from build123d import *

# Parameters (mm, degrees)
SKETCH1_W               = 24.51
SKETCH1_H               = 148
BOSS_EXTRUDE1_DEPTH     = 8
SKETCH2_W               = 8
SKETCH2_H               = 148
BOSS_EXTRUDE2_DEPTH     = 25
SKETCH4_W               = 20.3
SKETCH4_H               = 36.8
BOSS_EXTRUDE3_DEPTH     = 8
SKETCH5_W               = 23
SKETCH5_H               = 6
BOSS_EXTRUDE4_DEPTH     = 25
CUT_EXTRUDE2_REACH      = 151.752
SKETCH6_R               = 2
RIB1_REACH              = 159.03
SKETCH8_WALL_W          = 336.456302216
SKETCH8_WALL_H          = 3
MIRROR2_COPY_1_REACH    = 159.03
MIRROR2_COPY_1_SKETCH_W = 336.456302216
MIRROR2_COPY_1_SKETCH_H = 3
SKETCH3_R               = 2.5
CUT_EXTRUDE1_DEPTH      = 10
SKETCH12_R              = 2.75
CUT_EXTRUDE3_DEPTH      = 8
SKETCH13_W              = 5
SKETCH13_H              = 46
BOSS_EXTRUDE5_DEPTH     = 8
SKETCH14_W              = 3
SKETCH14_H              = 17
BOSS_EXTRUDE6_DEPTH     = 8
CHAMFER1_SIZE           = 2
CHAMFER2_SIZE           = 6
CHAMFER2_SIZE2          = 4.047051101
SKETCH15_W              = 33
SKETCH15_H              = 96
CUT_EXTRUDE4_DEPTH      = 45


with BuildPart() as part:
    # Sketch1 → Boss-Extrude1 (new body)
    with BuildSketch(Plane.XY):
        with Locations((-12.255, 74)):
            Rectangle(SKETCH1_W, SKETCH1_H)
    extrude(amount=BOSS_EXTRUDE1_DEPTH)

    # Sketch2 → Boss-Extrude2 (add)
    with BuildSketch(Plane.XY.offset(8)):
        with Locations((-20.51, 74)):
            Rectangle(SKETCH2_W, SKETCH2_H)
    extrude(amount=BOSS_EXTRUDE2_DEPTH)

    # Sketch4 → Boss-Extrude3 (add)
    with BuildSketch(Plane(origin=(0, 0, 0), x_dir=(-1, 0, 0), z_dir=(0, 0, -1))):
        with Locations((-10.15, 129.6)):
            Rectangle(SKETCH4_W, SKETCH4_H)
    extrude(amount=-BOSS_EXTRUDE3_DEPTH)

    # Sketch5 → Boss-Extrude4 (add)
    with BuildSketch(Plane.XY.offset(8)):
        with Locations((8.8, 118.2)):
            Rectangle(SKETCH5_W, SKETCH5_H)
        with Locations((8.8, 141)):
            Rectangle(SKETCH5_W, SKETCH5_H)
    extrude(amount=BOSS_EXTRUDE4_DEPTH)

    # Cut-Extrude2: up to this face of the body (flat: up to its plane)
    cut_extrude2_end = Plane(part.part.faces().sort_by_distance((8.8, 115.2, 20.5))[0])
    # Sketch6 → Cut-Extrude2 (cut, up to the picked face)
    with BuildSketch(Plane(origin=(0, 144, 0), x_dir=(1, 0, 0), z_dir=(0, 1, 0)), mode=Mode.PRIVATE) as cut_extrude2_sk1:
        with Locations(Location((6.6, -20.5, 0), (0, 0, 270))):
            Circle(SKETCH6_R)
    cut_extrude2_tool1 = split(extrude(cut_extrude2_sk1.sketch, amount=-CUT_EXTRUDE2_REACH, mode=Mode.PRIVATE), bisect_by=cut_extrude2_end, keep=Keep.BOTH, mode=Mode.PRIVATE)
    add(cut_extrude2_tool1.solids().sort_by(Axis((6.6, 144, 20.5), (0, -1, 0)))[0], mode=Mode.SUBTRACT)

    # Sketch8 wall → Rib1 (add, up to next)
    with BuildSketch(Plane(origin=(16.3, 146, 18), x_dir=(0, -0.196116135138, 0.980580675691), z_dir=(0, -0.980580675691, -0.196116135138)), mode=Mode.PRIVATE) as rib1_sk1:
        Rectangle(SKETCH8_WALL_W, SKETCH8_WALL_H)
    rib1_tool1 = extrude(rib1_sk1.sketch, amount=RIB1_REACH, mode=Mode.PRIVATE) - part.part
    rib1 = rib1_tool1.solids().sort_by_distance((16.3, 146, 18))[0]
    add(rib1)

    # Mirror1: Rib1 across plane
    add(rib1.mirror(Plane.ZX.offset(129.6)))

    # Mirror2: Rib1 across plane
    add(rib1.mirror(Plane.ZY.offset(-7.55)))

    # Mirror2 copy 1 sketch → Mirror2 copy 1 (add, up to next)
    with BuildSketch(Plane(origin=(-1.2, 113.2, 18), x_dir=(0, 0.196116135138, 0.980580675691), z_dir=(0, 0.980580675691, -0.196116135138)), mode=Mode.PRIVATE) as mirror2_copy_1_sk1:
        Rectangle(MIRROR2_COPY_1_SKETCH_W, MIRROR2_COPY_1_SKETCH_H)
    mirror2_copy_1_tool1 = extrude(mirror2_copy_1_sk1.sketch, amount=MIRROR2_COPY_1_REACH, mode=Mode.PRIVATE) - part.part
    add(mirror2_copy_1_tool1.solids().sort_by_distance((-1.2, 113.2, 18))[0])

    # Sketch3 → Cut-Extrude1 (cut)
    with BuildSketch(Plane.XY.offset(8)):
        with Locations((-8, 8)):
            Circle(SKETCH3_R)
        with Locations((-8, 40)):
            Circle(SKETCH3_R)
        with Locations((-8, 100)):
            Circle(SKETCH3_R)
        with Locations((-8, 132)):
            Circle(SKETCH3_R)
    extrude(amount=-CUT_EXTRUDE1_DEPTH, mode=Mode.SUBTRACT)

    # Sketch12 → Cut-Extrude3 (cut)
    with BuildSketch(Plane.ZY.offset(24.51)):
        with Locations((22, 138.8)):
            Circle(SKETCH12_R)
        with Locations((22, 106.8)):
            Circle(SKETCH12_R)
        with Locations((22, 41.7)):
            Circle(SKETCH12_R)
        with Locations((22, 9.7)):
            Circle(SKETCH12_R)
    extrude(amount=-CUT_EXTRUDE3_DEPTH, mode=Mode.SUBTRACT)

    # Sketch13 → Boss-Extrude5 (add)
    with BuildSketch(Plane(origin=(0, 0, 0), x_dir=(-1, 0, 0), z_dir=(0, 0, -1))):
        with Locations((-2.5, 23)):
            Rectangle(SKETCH13_W, SKETCH13_H)
    extrude(amount=-BOSS_EXTRUDE5_DEPTH)

    # Sketch14 → Boss-Extrude6 (add)
    with BuildSketch(Plane(origin=(0, 0, 0), x_dir=(-1, 0, 0), z_dir=(0, 0, -1))):
        with Locations((-1.5, 102.7)):
            Rectangle(SKETCH14_W, SKETCH14_H)
    extrude(amount=-BOSS_EXTRUDE6_DEPTH)

    # Chamfer1
    chamfer1_edges = [part.edges().sort_by_distance(p)[0] for p in [
        (0, 46, 4),
        (3, 111.2, 4),
        (0, 94.2, 4),
    ]]
    chamfer(chamfer1_edges, length=CHAMFER1_SIZE)

    # Chamfer2
    chamfer2_edges = [part.edges().sort_by_distance(p)[0] for p in [
        (8.8, 121.2, 8),
        (8.8, 138, 8),
    ]]
    chamfer2_side = [part.faces().sort_by_distance(p)[0] for p in [
        (-4.974591741, 76.782250606, 8),
    ]]
    chamfer(chamfer2_edges, length=CHAMFER2_SIZE, length2=CHAMFER2_SIZE2, reference=chamfer2_side[0])

    # Sketch15 → Cut-Extrude4 (cut)
    with BuildSketch(Plane(origin=(20.3, 0, 0), x_dir=(0, 0, -1), z_dir=(1, 0, 0))):
        with Locations((-16.5, 100)):
            Rectangle(SKETCH15_W, SKETCH15_H)
    extrude(amount=-CUT_EXTRUDE4_DEPTH, mode=Mode.SUBTRACT)


solid = part.part
Verification items for the finished model (mm, model axes). A direction names the side the tool comes from. Coordinates: 2 decimals unless noted, no trailing zeros. Order: outer loops, then holes, each group sorted by start corner. A loop starts at its lowest first (then second) coordinate and runs counter-clockwise, first axis right, second up. Notation, with made-up numbers: M 58,9 L 112,9 A23 cw 112,34 Z; hole C 78.25,-27.75 d6. An arc over 180 degrees is marked long. One line per item, written item: value. Start each with the question number.
Item 1: Scan lines: probe 1 along Y at (x, z) = (-8, 6.25); probe 2 along Z at (x, y) = (-19, 41.5); probe 3 along Y at (x, z) = (-19.5, 21). Record each from-to range of solid material in increasing order.
Item 2: Sectioned sample at B-B (z = 22). Enter the section's corners in (x, y).
Item 3: Sectioned sample at D-D (y = 47). Enter the section's corners in (x, z), then the cut area to 3 significant figures.
Item 4: Sectioned sample at C-C (x = -20). Enter the section's corners in (y, z).
Item 5: Access from +Z, -Z, +X, -X, +Y, -Y to the whole of each face (thin tool, end or side, straight path). Record for faces 1 (the flat face through (5, 23, 4)), 2 (the flat face through (-16.51, 26, 20)), 3 (the flat face through (0, 50, 4)).
Item 6: Sectioned sample at A-A (x = -8). Enter the section's corners in (y, z).
Item 7: Gauge pin test, flat ends, axial feed: pin 1 (3.5 mm diameter, centred on y = 41.7, z = 22, fed in from +X); pin 2 (6 mm diameter, centred on x = 1, y = 37.5, fed in from -Z); pin 3 (11 mm diameter, centred on x = -9.5, y = 36.5, fed in from +Z); pin 4 (4.5 mm diameter, centred on y = 49, z = 4.5, fed in from +X). Record the tip position at first contact, or that the pin passes through.
Item 8: Mould release check, pull along X, two halves, no side actions. Record for faces 4 (the flat face through (-6, 26, 8)), 5 (the cylindrical face through (-8.54, 5.56, 4.06)), 6 (the flat face through (1, 47, 4)): released by +X, released by -X, zero draft, split by the parting line, or undercut.
Conclusion:
1. probe 1: y = 0 to 5.5, 10.5 to 37.5, 42.5 to 52
1. probe 2: z = 0 to 19.26, 24.74 to 33
1. probe 3: y = 0 to 7.14, 12.26 to 39.14, 44.26 to 52
2. outline: M -24.51,0 L -16.51,0 L -16.51,6.95 L -24.51,6.95 Z; M -24.51,12.45 L -16.51,12.45 L -16.51,38.95 L -24.51,38.95 Z; M -24.51,44.45 L -16.51,44.45 L -16.51,52 L -24.51,52 Z
3. outline: M -24.51,0 L 1,0 L 1,8 L -16.51,8 L -16.51,33 L -24.51,33 Z
3. area: 404 mm^2
4. outline: M 0,0 L 52,0 L 52,33 L 0,33 Z; hole C 9.7,22 d5.5; hole C 41.7,22 d5.5
5. face 1: +Z, -Z, +X, +Y, -Y
5. face 2: +Z, +X, +Y, -Y
5. face 3: +Z, -Z, +X, +Y
6. outline: M 0,0 L 5.5,0 L 5.5,8 L 0,8 Z; M 10.5,0 L 37.5,0 L 37.5,8 L 10.5,8 Z; M 42.5,0 L 52,0 L 52,8 L 42.5,8 Z
7. pin 1: passes through
7. pin 2: stops at z = 0
7. pin 3: stops at z = 8
7. pin 4: stops at x = 1.25
8. face 4: zero draft
8. face 5: undercut
8. face 6: released by +X
